Here's how the part is built. I have some questions about the finished solid (model axes, mm). Give positions to 0.01 mm unless a question says otherwise; leave off trailing zeros. Loops run counter-clockwise (first coordinate to the right, second up) from the corner with the lowest first, then second, coordinate; pieces in that order, holes last.
Q1. If we section it at D-D (z = -16): Please give me the cut outline in (x, y).
Q2. Will these pins go through, and if not, where does the flat tip stop? P1, Ø1.3, axis at y = 1, z = -20.5, coming from the -X side; P2, Ø1.3, axis at x = 24.5, y = 1, coming from the -Z side; P3, Ø1.3, axis at y = 1, z = -20, coming from the +X side; P4, Ø3, axis at x = 0, z = 5, coming from the -Y side.
Q3. If we section it at B-B (z = 5): Please give me the cut outline in (x, y), plus the area to 3 significant figures.
Q4. I need wall thicknesses on line 1 (X direction, y = 1.1, z = 5); line 2 (X direction, y = 0.35, z = 3.5); line 3 (Z direction, x = 19, y = 1.2). Which ranges of each line are inside material? Lowest first, please.
Q5. If we section it at A-A (x = -20): Please give me the cut outline in (y, z).
Q6. If we section it at C-C (y = 0.55): Please give me the cut outline in (x, z).
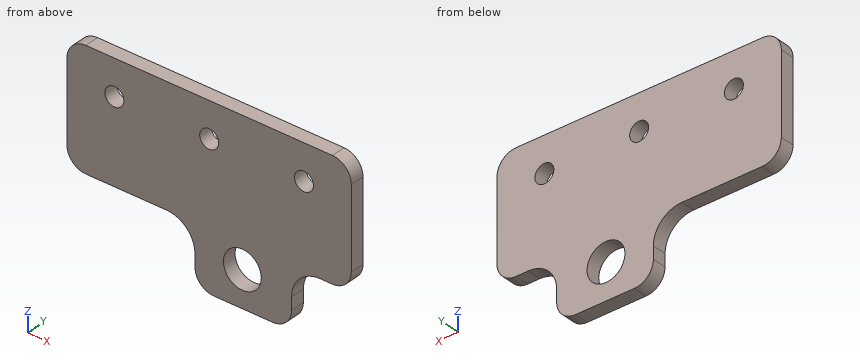
from build123d import *

# Parameters (mm, degrees)
SKETCH_1_W          = 60
SKETCH_1_H          = 25
SKETCH_1_R          = 2
EXTRUDE_1_DEPTH     = 3
SKETCH_2_R          = 4
CUT_EXTRUDE_1_DEPTH = 3
CUT_EXTRUDE_2_DEPTH = 10
FILLET_1_R          = 6
FILLET_2_R          = 4
FILLET_3_R          = 4


with BuildPart() as part:
    # 草图1 → 凸台-拉伸1 (new body)
    # profile 1 of 2: a face of its own
    with BuildSketch(Plane(origin=(0, 0, 0), x_dir=(1, 0, 0), z_dir=(0, 1, 0))):
        Rectangle(SKETCH_1_W, SKETCH_1_H)
        with Locations(Location((20, -5, 0), (0, 0, 270))):
            Circle(SKETCH_1_R, mode=Mode.SUBTRACT)
        with Locations(Location((-20, -5, 0), (0, 0, 270))):
            Circle(SKETCH_1_R, mode=Mode.SUBTRACT)
        with Locations(Location((0, -5, 0), (0, 0, 270))):
            Circle(SKETCH_1_R, mode=Mode.SUBTRACT)
    # profile 2 of 2: a face of its own
    with BuildSketch(Plane(origin=(0, 0, 0), x_dir=(1, 0, 0), z_dir=(0, 1, 0))):
        Polygon((10.919107028, 31.580892972), (30, 12.5), (-30, 12.5), align=None)
    extrude(amount=EXTRUDE_1_DEPTH)

    # 草图2 → 切除-拉伸1 (cut)
    with BuildSketch(Plane(origin=(0, 3, 0), x_dir=(1, 0, 0), z_dir=(0, 1, 0))):
        with Locations(Location((7, 17.5, 0), (0, 0, 270))):
            Circle(SKETCH_2_R)
    extrude(amount=-CUT_EXTRUDE_1_DEPTH, mode=Mode.SUBTRACT)

    # 草图3 → 切除-拉伸2 (cut)
    with BuildSketch(Plane(origin=(0, 3, 0), x_dir=(1, 0, 0), z_dir=(0, 1, 0))):
        Polygon((-3, 25.09030677), (-30, 12.5), (-3, 12.5), align=None)
        Polygon((10.919107028, 31.580892972), (-3, 25.09030677), (17.40969323, 25.09030677), align=None)
        Polygon((30, 12.5), (17.40969323, 25.09030677), (17.40969323, 12.5), align=None)
    extrude(amount=-CUT_EXTRUDE_2_DEPTH, mode=Mode.SUBTRACT)

    # 圆角1
    fillet_1_edges = [part.edges().sort_by_distance(p)[0] for p in [
        (-3, 1.5, -12.5),
        (17.40969323, 1.5, -12.5),
    ]]
    fillet(fillet_1_edges, radius=FILLET_1_R)

    # 圆角2
    fillet_2_edges = [part.edges().sort_by_distance(p)[0] for p in [
        (-3, 1.5, -25.09030677),
        (17.40969323, 1.5, -25.09030677),
    ]]
    fillet(fillet_2_edges, radius=FILLET_2_R)

    # 圆角3
    fillet_3_edges = [part.edges().sort_by_distance(p)[0] for p in [
        (30, 1.5, 12.5),
        (-30, 1.5, 12.5),
        (-30, 1.5, -12.5),
        (30, 1.5, -12.5),
    ]]
    fillet(fillet_3_edges, radius=FILLET_3_R)


solid = part.part
Check sheet entries:
1. outline: (-3.55, 0) - (3.29, 0) - (3.29, 3) - (-3.55, 3) - close; (10.71, 0) - (17.96, 0) - (17.96, 3) - (10.71, 3) - close
2. P1: stops at x = -3
2. P2: stops at z = -12.5
2. P3: stops at x = 17.41
2. P4: passes through
3. outline: (-30, 0) - (-22, 0) - (-22, 3) - (-30, 3) - close; (-18, 0) - (-2, 0) - (-2, 3) - (-18, 3) - close; (2, 0) - (18, 0) - (18, 3) - (2, 3) - close; (22, 0) - (30, 0) - (30, 3) - (22, 3) - close
3. area: 144 mm2
4. line 1: x = -30 to -22, -18 to -2, 2 to 18, 22 to 30
4. line 2: x = -30 to -21.32, -18.68 to -1.32, 1.32 to 18.68, 21.32 to 30
4. line 3: z = -14.43 to 3.27, 6.73 to 12.5
5. outline: (0, -12.5) - (3, -12.5) - (3, 3) - (0, 3) - close; (0, 7) - (3, 7) - (3, 12.5) - (0, 12.5) - close
6. outline: (-30, -8.5) arc R4 ccw to (-26, -12.5) - (-9, -12.5) arc R6 cw to (-3, -18.5) - (-3, -21.09) arc R4 ccw to (1, -25.09) - (13.41, -25.09) arc R4 ccw to (17.41, -21.09) - (17.41, -18.5) arc R6 cw to (23.41, -12.5) - (26, -12.5) arc R4 ccw to (30, -8.5) - (30, 8.5) arc R4 ccw to (26, 12.5) - (-26, 12.5) arc R4 ccw to (-30, 8.5) - close; hole circle Ø4 at (-20, 5); hole circle Ø4 at (0, 5); hole circle Ø8 at (7, -17.5); hole circle Ø4 at (20, 5)
